Autodesk Inventor part; units mm, degrees
ref_plane "YZ Plane" through (0, 0, 0) normal (1, 0, 0) x (0, 1, 0)
ref_plane "XZ Plane" through (0, 0, 0) normal (0, 1, 0) x (-1, 0, 0)
ref_plane "XY Plane" through (0, 0, 0) normal (0, 0, 1) x (1, 0, 0)
sketch "Sketch2" plane through (0, 0, 0) normal (0, 1, 0) x (-1, 0, 0)
  line L0 (0, 0) -> (155, 0)
  line L1 (155, 0) -> (155, -50)
  line L2 (155, -50) -> (0, -50)
  line L3 (0, -50) -> (0, 0)
  dimension "d4" = 155
  dimension "d5" = 50
extrude "Extrusion2" add sketch "Sketch2" along normal blind 35
sketch "Sketch4" plane through (0, 35, 0) normal (0, 1, 0) x (1, 0, 0)
  line L0 (0, 0) -> (0, 50)
  line L1 (0, 5) -> (-72, 5)
  line L2 (-72, 5) -> (-72, 45)
  line L3 (-72, 45) -> (0, 45)
  line L4 (0, 45) -> (0, 5)
  line L5 (-155, 50) -> (-155, 0) construction
  line L6 (-155, 25) -> (0, 25) construction
  dimension "d8" = 72
  dimension "d9" = 40
extrude "Extrusion3" cut sketch "Sketch4" against normal blind 26
sketch "Sketch5" plane through (0, 9, 0) normal (0, 1, 0) x (1, 0, 0)
  line L0 (0, 5) -> (-72, 5)
  line L1 (-72, 45) -> (0, 45)
  line L2 (0, 5) -> (-72, 5)
  line L3 (-72, 5) -> (-72, 23)
  line L4 (-72, 45) -> (0, 45)
  line L5 (0, 45) -> (0, 16.68)
  line L6 (-2, 8) -> (-70, 8)
  line L7 (-70, 8) -> (-70, 23)
  line L8 (-70, 42) -> (-2, 42)
  line L9 (-2, 42) -> (-2, 37)
  line L10 (0, 50) -> (0, 0) construction
  line L11 (0, 25) -> (-72, 25) construction
  line L12 (-72, 5) -> (-72, 45) construction
  line L13 (-36, 5) -> (-36, 42) construction
  line L14 (0, 45) -> (0, 5)
  line L15 (-2, 16.68) -> (0, 16.68)
  line L16 (0, 37) -> (-2, 37)
  line L17 (-2, 16.68) -> (-2, 8)
  line L18 (0, 16.68) -> (0, 5)
  line L19 (-72, 5) -> (-72, 45)
  line L20 (-70, 38) -> (-72, 38)
  line L21 (-72, 38) -> (-72, 23) construction
  line L22 (-72, 23) -> (-70, 23)
  line L23 (-70, 23) -> (-70, 25) construction
  line L24 (-70, 38) -> (-70, 42)
  line L25 (-70, 23) -> (-70, 38) construction
  line L26 (-72, 23) -> (-72, 38)
  line L27 (-72, 38) -> (-72, 45)
  dimension "d12" = 68
  dimension "d13" = 34
  dimension "d17" = 20.32
  dimension "d43" = 15
  dimension "d44" = 4
  dimension "d52" = 8
extrude "Extrusion5" add sketch "Sketch5" along normal blind 20 contours L0 L3 L22 L7 L6 L17 L15 L14 | L16 L9 L8 L24 L20 L19 L1 L5
fillet "Fillet2" radius 3 4 edges at (-2, 19, -8) (-70, 19, -8) (-70, 19, -42) (-2, 19, -42)
sketch "Sketch7" plane through (-155, 0, 0) normal (0, 0, 1) x (1, 0, 0)
  line L0 (89.9, 9) -> (104.9, 9)
  line L1 (104.9, 9) -> (104.9, 16)
  line L2 (104.9, 16) -> (89.9, 16)
  line L3 (89.9, 16) -> (89.9, 9)
  line L4 (89.9, 12.5) -> (104.9, 12.5) construction
  line L5 (97.4, 16) -> (97.4, 9) construction
  line L6 (88, 29) -> (88, 9) construction
  line L7 (88, 9) -> (150, 9) construction
  line L8 (85, 9) -> (85, 29)
  line L9 (120.4, 9) -> (132.4, 9)
  line L10 (132.4, 9) -> (132.4, 16) construction
  line L11 (132.4, 16) -> (120.4, 16)
  line L12 (120.4, 16) -> (120.4, 9)
  line L13 (133, 9) -> (145, 9)
  line L14 (145, 9) -> (145, 16)
  line L15 (145, 16) -> (133, 16)
  line L16 (133, 16) -> (133, 9) construction
  line L17 (126.4, 16) -> (126.4, 9) construction
  line L18 (139, 16) -> (139, 9) construction
  line L19 (132.4, 16) -> (133, 16) construction
  line L20 (132.4, 16) -> (133, 16)
  line L21 (132.4, 9) -> (133, 9)
  point P0 (155, 0)
  dimension "d29" = 15
  dimension "d30" = 7
  dimension "d32" = 0
  dimension "d35" = 12.4
  dimension "d36" = 12
  dimension "d37" = 7
  dimension "d38" = 12
  dimension "d39" = 7
  dimension "d40" = 41.4
  dimension "d41" = 54
extrude "Extrusion7" cut sketch "Sketch7" against normal up to next
sketch "Sketch9" plane through (0, 35, 0) normal (0, 1, 0) x (1, 0, 0)
  line L0 (-78, 44.5) -> (-150, 44.5)
  line L1 (-150, 44.5) -> (-150, 33.89)
  line L2 (-150, 5.5) -> (-78, 5.5)
  line L3 (-78, 5.5) -> (-78, 44.5)
  line L4 (0, 50) -> (0, 0) construction
  line L5 (0, 25) -> (-155, 25) construction
  line L6 (-155, 0) -> (-155, 50) construction
  line L7 (-150, 25) -> (-78, 25) construction
  line L8 (-155, 50) -> (-155, 0)
  line L9 (-150, 16.11) -> (-155, 16.11)
  line L10 (-155, 16.11) -> (-155, 33.89)
  line L11 (-155, 33.89) -> (-150, 33.89)
  line L12 (-150, 33.89) -> (-150, 25) construction
  line L13 (-150, 25) -> (-155, 25) construction
  line L14 (-150, 33.89) -> (-150, 25) construction
  line L15 (-150, 16.11) -> (-150, 5.5)
  line L16 (-150, 25) -> (-150, 16.11) construction
  line L17 (-150, 25) -> (-150, 16.11) construction
  dimension "d45" = 72
  dimension "d46" = 39
  dimension "d47" = 5
  dimension "d50" = 17.78
extrude "Extrusion8" cut sketch "Sketch9" against normal blind 30
fillet "Fillet3" radius 10 4 edges at (0, 17.5, 0) (0, 17.5, -50) (-155, 17.5, 0) (-155, 17.5, -50)
chamfer "Chamfer1" distance 8.89 angle 45 2 edges at (-152.5, 5, -33.89) (-152.5, 5, -16.11)
equation "\"d37\" = d30"
equation "\"d38\" = d36"
equation "\"d39\" = d37"
properties part number "PiHolder"
CAD build for the part. Positions are in the model's coordinates, mm. A direction names the side the tool comes from. Coordinates: 2 decimals unless noted, no trailing zeros. Write each loop counter-clockwise with the first axis right and the second up, starting at its lowest first coordinate (ties: lowest second). Pieces come first, ordered by that corner, then holes. Notation, with made-up numbers: (72.25, 82.5) - (130.25, 82.5) arc R17 cw to (130.25, 104.5) - close; hole circle Ø5 at (41, -4.5). An arc over 180 degrees is marked (long way). Use a Markdown table: item, result. Add a question column.
Item 1: Drill centre lines: L1, parallel to Z at x = -71, y = 33.5; L2, parallel to Z at x = -50.5, y = 26; L3, parallel to X at y = 31, z = -14. Where is each one in solid material? Low to high. Write a range as from..to.
Item 2: Flat gauge pins, fed straight in: pin 1 (3.5 mm diameter, centred on y = 12, z = -3.5, fed in from +X); pin 2 (12 mm diameter, centred on y = 27, z = -26, fed in from +X); pin 3 (1.6 mm diameter, centred on x = -1, y = 15, fed in from -Z). Where does each tip first touch, or does it go through?
Item 3: 3-axis set-ups, long thin cutter, end or side, ignore diameter. For faces 5 (the face through (-57, 16, -4)), 6 (the face through (-69.1, 19.14, -41.14)), 7 (the face through (-155, 9, -31)), 8 (the face through (-36, 29, -43)), 9 (the face through (-77, 17, 0)): which of +Z, -Z, +X, -X, +Y, -Y reach the whole face in a straight line?
Item 4: Band-saw the part on A-A, the plane x = -57.5. Give the cut face in (y, z).
Item 5: Mould opens along Z. For faces 1 (the face through (-2.85, 17.74, -46.99)), 2 (the face through (-37, 9, -21)), 3 (the face through (0, 8, -25)), 4 (the face through (-150, 20, -11)) say: pulls with the +Z half, pulls with the -Z half, needs draft (parallel to the pull), parting line crosses it, or undercut.
Item 6: Band-saw the part on C-C, the plane x = -100.5. Give the cut face in (y, z), and give its area (3 significant figures).
Item 7: Band-saw the part on D-D, the plane z = -32.5. Give the cut face in (x, y), and give its area (3 significant figures).
Numbers:
| question | item | result |
|---|---|---|
| 1 | L1 | -50..-45, -5..0 |
| 1 | L2 | -50..-42, -8..0 |
| 1 | L3 | -155..-150, -78..-72 |
| 2 | pin 1 | x = -1.2 |
| 2 | pin 2 | x = -70 |
| 2 | pin 3 | z = -45.72 |
| 3 | face 5 | +Z |
| 3 | face 6 | +Y |
| 3 | face 7 | +Z, -Z, -X, +Y, -Y |
| 3 | face 8 | +X, +Y |
| 3 | face 9 | +Z, +X, -X, +Y, -Y |
| 4 | outline | (0, -50) - (35, -50) - (35, -45) - (29, -45) - (29, -42) - (9, -42) - (9, 0) - (0, 0) - close; (16, -8) - (29, -8) - (29, -5) - (35, -5) - (35, 0) - (16, 0) - close |
| 5 | face 1 | pulls with the -Z half |
| 5 | face 2 | undercut |
| 5 | face 3 | needs draft |
| 5 | face 4 | undercut |
| 6 | outline | (0, -50) - (35, -50) - (35, -44.5) - (5, -44.5) - (5, -5.5) - (35, -5.5) - (35, 0) - (0, 0) - close |
| 6 | area | 580 mm2 |
| 7 | outline | (-155, 0) - (0, 0) - (0, 9) - (-72, 9) - (-72, 35) - (-78, 35) - (-78, 5) - (-150, 5) - (-150, 12.5) - (-155, 12.5) - close |
| 7 | area | 1,280 mm2 |
